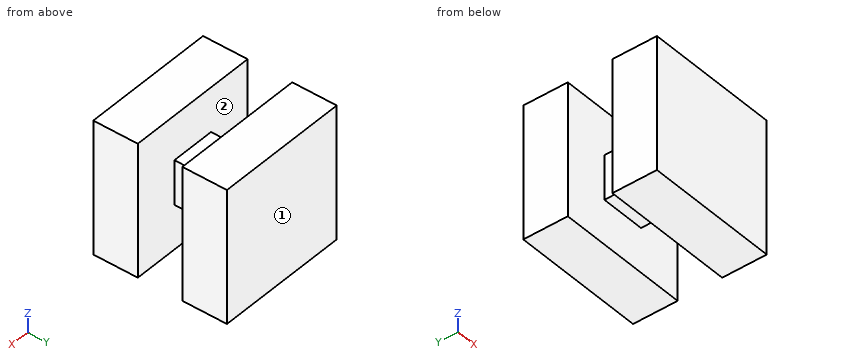
```python
from build123d import *

# Parameters (mm, degrees)
SKETCH1_W           = 60
SKETCH1_H           = 60
BOSS_EXTRUDE1_DEPTH = 60
SKETCH2_W           = 20
SKETCH2_H           = 20
CUT_EXTRUDE1_DEPTH  = 60
SKETCH3_W           = 20
SKETCH3_H           = 20
CUT_EXTRUDE2_DEPTH  = 20
SKETCH4_W           = 20
SKETCH4_H           = 20
CUT_EXTRUDE3_DEPTH  = 20
SKETCH5_W           = 20
SKETCH5_H           = 20
BOSS_EXTRUDE2_DEPTH = 20


with BuildPart() as part:
    # Sketch1 → Boss-Extrude1 (new body)
    with BuildSketch(Plane.XY):
        with Locations((30, 30)):
            Rectangle(SKETCH1_W, SKETCH1_H)
    extrude(amount=BOSS_EXTRUDE1_DEPTH)

    # Sketch2 → Cut-Extrude1 (cut)
    with BuildSketch(Plane.XY.offset(60)):
        with Locations((10, 30)):
            Rectangle(SKETCH2_W, SKETCH2_H)
        with Locations((50, 30)):
            Rectangle(SKETCH2_W, SKETCH2_H)
    extrude(amount=-CUT_EXTRUDE1_DEPTH, mode=Mode.SUBTRACT)

    # Sketch3 → Cut-Extrude2 (cut)
    with BuildSketch(Plane.ZY):
        with Locations((30, 50)):
            Rectangle(SKETCH3_W, SKETCH3_H)
        with Locations((30, 10)):
            Rectangle(SKETCH3_W, SKETCH3_H)
    extrude(amount=-CUT_EXTRUDE2_DEPTH, mode=Mode.SUBTRACT)

    # Sketch4 → Cut-Extrude3 (cut)
    with BuildSketch(Plane.ZY.offset(-20)):
        with Locations((10, 30)):
            Rectangle(SKETCH4_W, SKETCH4_H)
        with Locations((50, 30)):
            Rectangle(SKETCH4_W, SKETCH4_H)
    extrude(amount=-CUT_EXTRUDE3_DEPTH, mode=Mode.SUBTRACT)

    # Sketch5 → Boss-Extrude2 (add)
    with BuildSketch(Plane.ZY.offset(-20)):
        with Locations((30, 50)):
            Rectangle(SKETCH5_W, SKETCH5_H)
        with Locations((30, 10)):
            Rectangle(SKETCH5_W, SKETCH5_H)
    extrude(amount=BOSS_EXTRUDE2_DEPTH)


solid = part.part
```
Input: part model. Units: mm. Frame: model coordinates. Face numbers are marked on the shaded views. A direction names the side the tool comes from. Coordinates: 2 decimals unless noted, no trailing zeros. Loops run counter-clockwise (first coordinate to the right, second up) from the corner with the lowest first, then second, coordinate; pieces in that order, holes last. Notation, with made-up numbers: M -10.5,-6 L 20.5,-6 A9 cw 20.5,-1 Z; hole C -38.75,-20 d10. An arc over 180 degrees is marked long. Answer in a Markdown table with one row per item.
1. First-contact query: pin 1 (1.5 mm diameter, centred on x = 51, z = 9.5, fed in from -Y); pin 2 (10 mm diameter, centred on x = 35, y = 26, fed in from +Z); pin 3 (6 mm diameter, centred on y = 33, z = 28.5, fed in from -X); pin 4 (16 mm diameter, centred on y = 31, z = 29.5, fed in from +X). Flat tips, straight axial feed; report the tip coordinate or a pass-through.
Response:
| item | result |
|---|---|
| pin 1 | stops at y = 0 |
| pin 2 | stops at z = 40 |
| pin 3 | stops at x = 20 |
| pin 4 | stops at x = 40 |
2. Reachability of the marked faces 1 and 2 from +Z, -Z, +X, -X, +Y, -Y: full face, straight path, thin tool, end or side. Return the list, or none.
Response:
| item | result |
|---|---|
| face 1 | +Z, -Z, +X, -X, +Y |
| face 2 | none |
3. Section B-B, the plane z = 54. Output: boundary loops of the cut face in (x, y), then the cut area to 3 significant figures.
Response:
| item | result |
|---|---|
| outline | M 0,0 L 60,0 L 60,20 L 0,20 Z; M 0,40 L 60,40 L 60,60 L 0,60 Z |
| area | 2,400 mm2 |
4. Section C-C, the plane x = 21. Output: boundary loops of the cut face in (y, z).
Response:
| item | result |
|---|---|
| outline | M 0,0 L 20,0 L 20,20 L 40,20 L 40,0 L 60,0 L 60,60 L 40,60 L 40,40 L 20,40 L 20,60 L 0,60 Z |
5. Section A-A, the plane x = 7. Output: boundary loops of the cut face in (y, z), then the cut area to 3 significant figures.
Response:
| item | result |
|---|---|
| outline | M 0,0 L 20,0 L 20,60 L 0,60 Z; M 40,0 L 60,0 L 60,60 L 40,60 Z |
| area | 2,400 mm2 |
6. Section D-D, the plane z = 33.5. Output: boundary loops of the cut face in (x, y).
Response:
| item | result |
|---|---|
| outline | M 0,0 L 60,0 L 60,20 L 40,20 L 40,40 L 60,40 L 60,60 L 0,60 L 0,40 L 20,40 L 20,20 L 0,20 Z |
7. Material intervals for line 1 (Y direction, x = 15, z = 5.5); line 2 (Z direction, x = 22.5, y = 25.5), sorted ascending.
Response:
| item | result |
|---|---|
| line 1 | y = 0 to 20, 40 to 60 |
| line 2 | z = 20 to 40 |
